Geometry: final body of the model. Coordinates: model frame, mm. Coordinates: 2 decimals unless noted, no trailing zeros. Loops run counter-clockwise (first coordinate to the right, second up) from the corner with the lowest first, then second, coordinate; pieces in that order, holes last. Notation, with made-up numbers: M 50,43 L 55,43 A29 ccw 55,65 Z; hole C 17.25,72 d2. An arc over 180 degrees is marked long. Write each question's results on one line, items separated by ' | '. Start each with the question number.
from build123d import *

# Parameters (mm, degrees)
CROQUIS1_R              = 107.5
SALIENTE_EXTRUIR1_DEPTH = 10
MATRIZC1_COUNT          = 6
CROQUIS4_R              = 55
CORTAR_EXTRUIR1_DEPTH   = 10


with BuildPart() as part:
    # Croquis1 → Saliente-Extruir1 (new body)
    with BuildSketch(Plane(origin=(0, 0, 0), x_dir=(1, 0, 0), z_dir=(0, 1, 0))):
        with Locations(Location((0, 0, 0), (0, 0, 270))):
            Circle(CROQUIS1_R)
    extrude(amount=SALIENTE_EXTRUIR1_DEPTH)

    # Croquis6 → Taladro de margen para M121 (revolve, cut)
    with BuildSketch(Plane(origin=(0, 10, -97.5), x_dir=(0, 0, 1), z_dir=(1, 0, 0))):
        Polygon((0, 0), (0, 47.555809178), (6.75, 43.5), (6.75, 0), align=None)
    taladro_de_margen_para_m121 = revolve(axis=Axis((0, 16.35, -97.5), (0, -1, 0)), mode=Mode.SUBTRACT)

    # MatrizC1: Taladro de margen para M121 ×6 about axis
    matrizc1_axis = Axis((0, 0, 0.385932096), (0, 1, 0))
    for i in range(1, MATRIZC1_COUNT):
        add(taladro_de_margen_para_m121.rotate(matrizc1_axis, i * 360 / MATRIZC1_COUNT), mode=Mode.SUBTRACT)

    # Croquis4 → Cortar-Extruir1 (cut)
    with BuildSketch(Plane(origin=(0, 10, 0), x_dir=(1, 0, 0), z_dir=(0, 1, 0))):
        with Locations(Location((0, 0, 0), (0, 0, 270))):
            Circle(CROQUIS4_R)
    extrude(amount=-CORTAR_EXTRUIR1_DEPTH, mode=Mode.SUBTRACT)


solid = part.part
Item 1: Section B-B, the plane x = 0. Return loops of the section in (y, z), plus the area to 3 significant figures.
Item 2: Ray query, L1, parallel to Z at x = 86, y = 0.75; L2, parallel to X at y = 4.25, z = 0.5; L3, parallel to X at y = 8, z = -32.5. Return the intervals inside material, ascending. Write a range as [from, to].
Item 3: Pull-direction query (Z, two-part tool) for faces 1 (the flat face through (25.4, 10, -49.3)), 2 (the cylindrical face through (-104.944, 4.93, -23.304)), 3 (the cylindrical face through (-82.186, 5.07, 55.564)); classes: released by +Z, released by -Z, zero draft, split by the parting line, or undercut.
Item 4: Section A-A, the plane z = 0. Return loops of the section in (x, y).
Item 5: Contact query for flat-ended pins moving along their axis: P1, Ø4, axis at y = 5, z = 7, coming from the +X side; P2, Ø6, axis at x = 24.5, y = 5, coming from the +Z side. Output: stop coordinate, or through.
Item 6: Section C-C, the plane x = -88. Return loops of the section in (y, z).
Item 7: Section D-D, the plane y = 3. Return loops of the section in (x, z), plus the area to 3 significant figures.
Solutions:
1) outline: M 0,-107.5 L 10,-107.5 L 10,-104.25 L 0,-104.25 Z; M 0,-90.75 L 10,-90.75 L 10,-55 L 0,-55 Z; M 0,55 L 10,55 L 10,91.52 L 0,91.52 Z; M 0,105.02 L 10,105.02 L 10,107.5 L 0,107.5 Z | area: 780 mm²
2) L1: z = [-64.5, -55.19], [-41.92, 42.69], [55.97, 64.5] | L2: x = [-107.5, -55], [55, 107.5] | L3: x = [-102.47, -44.37], [44.37, 102.47]
3) face 1: zero draft | face 2: split by the parting line | face 3: undercut
4) outline: M -107.5,0 L -55,0 L -55,10 L -107.5,10 Z; M 55,0 L 107.5,0 L 107.5,10 L 55,10 Z
5) P1: stops at x = 107.38 | P2: stops at z = 105.33
6) outline: M 0,-61.74 L 10,-61.74 L 10,-54.48 L 0,-54.48 Z; M 0,-42.63 L 10,-42.63 L 10,43.4 L 0,43.4 Z; M 0,55.26 L 10,55.26 L 10,61.74 L 0,61.74 Z
7) outline: C 0,0 d215; hole C -84.77,-48.56 d13.5; hole C -84.77,49.33 d13.5; hole C 0,0 d110; hole C 0,-97.5 d13.5; hole C 0,98.27 d13.5; hole C 84.77,-48.56 d13.5; hole C 84.77,49.33 d13.5 | area: 25,900 mm²
